The model under review builds one solid part; all positions refer to its coordinate system, in mm. A direction names the side the tool comes from. Round coordinates to 2 decimals unless told otherwise and drop trailing zeros. Write each loop counter-clockwise with the first axis right and the second up, starting at its lowest first coordinate (ties: lowest second). Pieces come first, ordered by that corner, then holes. Notation, with made-up numbers: (82, 76) - (112, 76) arc R22 ccw to (112, 89) - close; hole circle Ø11 at (81, 76). An arc over 180 degrees is marked (long way). Use one line per item in the form item = value.
from build123d import *

# Parameters (mm, degrees)
BOSS_EXTRUDE1_DEPTH = 50
SKETCH3_R           = 10
CUT_EXTRUDE1_DEPTH  = 1234.101799213


with BuildPart() as part:
    # Sketch1 → Boss-Extrude1 (new body)
    with BuildSketch(Plane.XY):
        with BuildLine():
            Line((-546.37161216, -857.105521629), (-539.348809346, -864.224527221))
            ThreePointArc((-539.348809346, -864.224527221), (-580.373107294, -775.216346142), (-605.714285714, -869.890915047))
            ThreePointArc((-605.714285714, -869.890915047), (0, -1060), (605.714285714, -869.890915047))
            ThreePointArc((605.714285714, -869.890915047), (580.373107294, -775.216346142), (539.348809346, -864.224527221))
            Line((539.348809346, -864.224527221), (546.37161216, -857.105521629))
            ThreePointArc((546.37161216, -857.105521629), (579.522386954, -785.180094177), (600, -861.684396981))
            ThreePointArc((600, -861.684396981), (0, -1050), (-600, -861.684396981))
            ThreePointArc((-600, -861.684396981), (-579.522386954, -785.180094177), (-546.37161216, -857.105521629))
        make_face()
    extrude(amount=BOSS_EXTRUDE1_DEPTH)

    # Sketch3 → Cut-Extrude1 (cut, through all)
    with BuildSketch(Plane(origin=(0, 0, 0), x_dir=(1, 0, 0), z_dir=(0, 1, 0))):
        with Locations(Location((0, -22.5, 0), (0, 0, 270))):
            Circle(SKETCH3_R)
    extrude(amount=-CUT_EXTRUDE1_DEPTH, mode=Mode.SUBTRACT)


solid = part.part
(1) Insertion check: P1, Ø12, axis at x = 0, z = 22.5, coming from the -Y side; P2, Ø5, axis at x = 230, z = 40.5, coming from the +Y side; P3, Ø1, axis at x = -242, z = 17.5, coming from the -Y side; P4, Ø10, axis at x = -168.5, z = 7.5, coming from the -Y side. Each pin has a flat end and moves straight along its axis. Give the tip position at first contact, or say it passes through.
Geometry results:
P1 = through
P2 = -1023.94
P3 = -1032.12
P4 = -1047.31
(2) The part is to be moulded in two halves that separate along X. For faces 3 (the cylindrical face through (-9.03, -1059.96, 30.21)), 4 (the cylindrical face through (578.08, -785.08, 24.65)), 5 (the flat face through (-3, -1054, 0)), say which applies: +X half, -X half, draft (parallel to the pull), parting line (faces both ways), or undercut.
Geometry results:
face_3 = parting line
face_4 = undercut
face_5 = draft
(3) To check wall thickness, follow L1, parallel to Z at x = 0, y = -1055; L2, parallel to X at y = -819, z = 42; L3, parallel to X at y = -812, z = 20. State the ranges of each line that lie inside material, in increasing order.
Geometry results:
L1 = 0 to 12.5, 32.5 to 50
L2 = -627.41 to -617.25, -534.63 to -524.47, 524.47 to 534.63, 617.25 to 627.41
L3 = -625.8 to -615.23, -536.65 to -526.08, 526.08 to 536.65, 615.23 to 625.8
(4) Add section D-D on x = -161. Write out the cut boundary in (y, z), then the cut area to 3 significant figures.
Geometry results:
outline = (-1047.7, 0) - (-1037.58, 0) - (-1037.58, 50) - (-1047.7, 50) - close
area = 506 mm2
(5) Machinability: for faces 1 (the cylindrical face through (8.94, -1049.96, 30.21)), 2 (the cylindrical face through (3, -1054.91, 32.04)), which of the approach directions +Z, -Z, +X, -X, +Y, -Y give a long, thin tool a straight path to every point of the face, cutting with its end or side? Answer none if there is none.
Geometry results:
face_1 = +Z, -Z
face_2 = +Y, -Y
(6) Add section A-A on y = -797. Write out the cut boundary in (x, z), then the cut area to 3 significant figures.
Geometry results:
outline = (-618.45, 0) - (-605.35, 0) - (-605.35, 50) - (-618.45, 50) - close; (-546.53, 0) - (-533.43, 0) - (-533.43, 50) - (-546.53, 50) - close; (533.43, 0) - (546.53, 0) - (546.53, 50) - (533.43, 50) - close; (605.35, 0) - (618.45, 0) - (618.45, 50) - (605.35, 50) - close
area = 2,620 mm2
(7) Add section B-B on z = 22.5. Write out the cut boundary in (x, y), then the cut area to 3 significant figures.
Geometry results:
outline = (-605.71, -869.89) arc R1060 ccw to (-10, -1059.95) - (-10, -1049.95) arc R1050 cw to (-600, -861.68) arc R42.1 cw (long way) to (-546.37, -857.11) - (-539.35, -864.22) arc R52.1 ccw (long way) to start; (10, -1059.95) arc R1060 ccw to (605.71, -869.89) arc R52.1 ccw (long way) to (539.35, -864.22) - (546.37, -857.11) arc R42.1 cw (long way) to (600, -861.68) arc R1050 cw to (10, -1049.95) - close
area = 17,200 mm2
